Work out the finished part from the listing and answer in its coordinate system (mm). A direction names the side the tool comes from. Coordinates: 2 decimals unless noted, no trailing zeros. Loops run counter-clockwise (first coordinate to the right, second up) from the corner with the lowest first, then second, coordinate; pieces in that order, holes last. Notation, with made-up numbers: (73.5, 76) -> (97.5, 76) arc R31 cw to (97.5, 115) -> close; hole circle Ø6 at (46, 15.5). An arc over 180 degrees is marked (long way). One line per question, with ' | ' between items.
```python
from build123d import *
from OCP.BRepFilletAPI import BRepFilletAPI_MakeChamfer

# Parameters (mm, degrees)
RESSALTO_EXTRUS_O1_DEPTH = 5
ESBO_O2_R                = 1
CORTE_EXTRUS_O1_DEPTH    = 35.84250278
CORTE_EXTRUS_O2_DEPTH    = 2
SKETCH1_R                = 0.5
CUT_EXTRUDE1_DEPTH       = 20.931131428
SKETCH2_W                = 7
SKETCH2_H                = 3
BOSS_EXTRUDE1_DEPTH      = 4.2
SKETCH3_R                = 1.5
CUT_EXTRUDE2_DEPTH       = 23.33584563
FILLET2_R                = 3.5
CHAMFER1_SIZE            = 3
CHAMFER1_SIZE2           = 1.732050808


with BuildPart() as part:
    # Esboço1 → Ressalto-extrusão1 (new body)
    with BuildSketch(Plane.XY):
        Polygon((9, -10), (16.5, -10), (16.5, 10), (-16.5, 10), (-16.5, -10), (-6, -10), (-6, -5), (9, -5), align=None)
    extrude(amount=RESSALTO_EXTRUS_O1_DEPTH)

    # Esboço2 → Corte-extrusão1 (cut, through all)
    with BuildSketch(Plane(origin=(16.5, 0, 0), x_dir=(0, 0, -1), z_dir=(1, 0, 0))):
        with Locations((-2.5, -7.5)):
            Circle(ESBO_O2_R)
    extrude(amount=-CORTE_EXTRUS_O1_DEPTH, mode=Mode.SUBTRACT)

    # Esboço3 → Corte-extrusão2 (cut)
    with BuildSketch(Plane.XY.offset(5)):
        with BuildLine():
            Line((-16.5, 10), (-16.5, -1.963769034))
            ThreePointArc((-16.5, -1.963769034), (-0.129411774, 1.783536996), (16.5, 4.128984796))
            Line((16.5, 4.128984796), (16.5, 5.523404181))
            Line((16.5, 5.523404181), (16.5, 10))
            Line((16.5, 10), (-16.5, 10))
        make_face()
    extrude(amount=-CORTE_EXTRUS_O2_DEPTH, mode=Mode.SUBTRACT)

    # Sketch1 → Cut-Extrude1 (cut, through all)
    with BuildSketch(Plane(origin=(0, 0, 0), x_dir=(-1, 0, 0), z_dir=(0, 0, -1))):
        with Locations(Location((-11.5, 7, 0), (0, 0, 180))):
            Circle(SKETCH1_R)
    extrude(amount=-CUT_EXTRUDE1_DEPTH, mode=Mode.SUBTRACT)

    # Sketch2 → Boss-Extrude1 (add)
    with BuildSketch(Plane(origin=(0, 10, 0), x_dir=(1, 0, 0), z_dir=(0, 1, 0))):
        with Locations((-13, -1.5)):
            Rectangle(SKETCH2_W, SKETCH2_H)
    extrude(amount=BOSS_EXTRUDE1_DEPTH)

    # Sketch3 → Cut-Extrude2 (cut, through all)
    with BuildSketch(Plane(origin=(0, 0, 0), x_dir=(-1, 0, 0), z_dir=(0, 0, -1))):
        with Locations((13, 10.7)):
            Circle(SKETCH3_R)
    extrude(amount=-CUT_EXTRUDE2_DEPTH, mode=Mode.SUBTRACT)

    # Fillet2
    fillet2_edges = [part.edges().sort_by_distance(p)[0] for p in [
        (-9.5, 14.2, 1.5),
        (-16.5, 14.2, 1.5),
    ]]
    fillet(fillet2_edges, radius=FILLET2_R - 0.0001)  # a hair under: the kernel refuses the full size

    # Chamfer1: one chamfer whose edges measure the first distance from different faces: ONE call of the kernel's chamfer builder (chamfer() names one face for all edges)
    chamfer1_edges_1 = [part.edges().sort_by_distance(p)[0] for p in [
        (-11.25, -10, 5),
    ]]
    chamfer1_side_1 = [part.faces().sort_by_distance(p)[0] for p in [
        (-11.25, -10, 2.5),
    ]]
    chamfer1_edges_2 = [part.edges().sort_by_distance(p)[0] for p in [
        (12.75, -10, 5),
    ]]
    chamfer1_side_2 = [part.faces().sort_by_distance(p)[0] for p in [
        (12.75, -10, 2.5),
    ]]
    chamfer1 = BRepFilletAPI_MakeChamfer(part.part.solid().wrapped)
    for e in chamfer1_edges_1:
        chamfer1.Add(CHAMFER1_SIZE, CHAMFER1_SIZE2, e.wrapped, chamfer1_side_1[0].wrapped)  # the first distance lies on this face
    for e in chamfer1_edges_2:
        chamfer1.Add(CHAMFER1_SIZE, CHAMFER1_SIZE2, e.wrapped, chamfer1_side_2[0].wrapped)  # the first distance lies on this face
    add(Compound.cast(chamfer1.Shape()), mode=Mode.REPLACE)


solid = part.part
```
1) Find the intervals of material crossed by line 1 along Y through (x, z) = (-13, 0.95); line 2 along Y through (x, z) = (11.5, 0.85); line 3 along X through (y, z) = (-8.5, 3.7), in increasing order.
Check values:
line 1: y = -10 to 9.2, 12.2 to 14.2 | line 2: y = -10 to 6.5, 7.5 to 10 | line 3: x = -16.5 to -6, 9 to 16.5
2) The mould has two halves that part along Z. Classify faces 1 (the face through (-11.324, -9.122, 3.521)), 2 (the face through (12.8, -6.51, 2.63)), 3 (the face through (4, 10, 1)), 4 (the face through (-11.18, -6.51, 2.63)): released by +Z, released by -Z, zero draft, split by the parting line, or undercut.
Check values:
face 1: released by +Z | face 2: undercut | face 3: zero draft | face 4: undercut
3) Find section C-C (y = 7). Write down the section's boundary in (x, z), plus the area to 3 significant figures.
Check values:
outline: (-16.5, 0) -> (11, 0) -> (11, 3) -> (-16.5, 3) -> close; (12, 0) -> (16.5, 0) -> (16.5, 3) -> (12, 3) -> close | area: 96.0 mm^2
4) Find section D-D (x = 11.5). Write down the section's boundary in (y, z), plus the area to 3 significant figures.
Check values:
outline: (-10, 0) -> (6.5, 0) -> (6.5, 3) -> (3.57, 3) -> (3.57, 5) -> (-8.27, 5) -> (-10, 2) -> close; (7.5, 0) -> (10, 0) -> (10, 3) -> (7.5, 3) -> close; hole circle Ø2 at (-7.5, 2.5) | area: 78.4 mm^2
5) Flat-ended cylindrical pins translate along their axes: pin 1 (13 mm diameter, centred on x = -8, y = 7.5, fed in from +Z); pin 2 (1.5 mm diameter, centred on x = -11.5, z = 2.5, fed in from +Y). Find the tip coordinate at first contact, or state that the pin passes through.
Check values:
pin 1: stops at z = 3 | pin 2: stops at y = 14.12
6) Find section A-A (y = -7.5). Write down the section's boundary in (x, z), plus the area to 3 significant figures.
Check values:
outline: (-16.5, 0) -> (-6, 0) -> (-6, 1.5) -> (-16.5, 1.5) -> close; (-16.5, 3.5) -> (-6, 3.5) -> (-6, 5) -> (-16.5, 5) -> close; (9, 0) -> (16.5, 0) -> (16.5, 1.5) -> (9, 1.5) -> close; (9, 3.5) -> (16.5, 3.5) -> (16.5, 5) -> (9, 5) -> close | area: 54.0 mm^2
7) Find section B-B (z = 0.6). State how many separate pieces and enclosed holes the cut face has, plus the area to 3 significant figures.
Check values:
separate pieces: 1 | enclosed holes: 2 | area: 601 mm^2
8) For faces 5 (the face through (16.5, 0, 2)), 6 (the face through (1, -5, 2)), 7 (the face through (-4, 6, 3)), determine the directions among +Z, -Z, +X, -X, +Y, -Y from which every point of the face is accessible in a straight line to the end or side of a thin tool.
Check values:
face 5: +Z, -Z, +X, +Y, -Y | face 6: +Z, -Z, -Y | face 7: +Z, -X, +Y
